from build123d import *

# Parameters (mm, degrees)
EXTRUDE_2_DEPTH = 36


with BuildPart() as part:
    # Эскиз2 → Повернуть1 (revolve)
    with BuildSketch(Plane(origin=(0, 0, 0), x_dir=(1, 0, 0), z_dir=(0, 1, 0))):
        with BuildLine():
            Line((-18, 25), (-18, 0))
            Line((-18, 0), (-20.75, 0))
            Line((-20.75, 0), (-20.75, -2.75))
            Line((-20.75, -2.75), (-18, -2.75))
            Line((-18, -2.75), (-18, -5.5))
            Line((-18, -5.5), (-20.75, -5.5))
            Line((-20.75, -5.5), (-20.75, -8.25))
            Line((-20.75, -8.25), (-18.916666667, -8.25))
            Line((-18.916666667, -8.25), (-18.916666667, -11))
            Line((-18.916666667, -11), (-22, -11))
            ThreePointArc((-22, -11), (-25.889087297, -9.389087297), (-27.5, -5.5))
            Line((-27.5, -5.5), (-27.5, 0))
            Line((-27.5, 0), (-30.395, 2.895))
            Line((-30.395, 2.895), (-30.395, 22.105))
            Line((-30.395, 22.105), (-27.5, 25))
            Line((-27.5, 25), (-18, 25))
        make_face()
    revolve(axis=Axis((0, 0, 84.230364838), (0, 0, -1)))


with BuildPart() as body_2:
    # Эскиз3 → Бобышка-Вытянуть2 (new body)
    with BuildSketch(Plane(origin=(0, 0, -25), x_dir=(-1, 0, 0), z_dir=(0, 0, -1))):
        Polygon((0, -31.754264805), (27.5, -15.877132403), (27.5, 15.877132403), (0, 31.754264805), (-27.5, 15.877132403), (-27.5, -15.877132403), align=None)
    extrude(amount=-EXTRUDE_2_DEPTH)


with BuildPart() as part_1:
    add(part.part)

    # Combine 1: intersect body 2
    add(body_2.part, mode=Mode.INTERSECT)


solid = part_1.part
Source: CAD feature listing. Evaluate the final solid. Frame: model axes, mm. A direction names the side the tool comes from. Give positions to 0.01 mm unless a question says otherwise; leave off trailing zeros. Write each loop counter-clockwise with the first axis right and the second up, starting at its lowest first coordinate (ties: lowest second). Pieces come first, ordered by that corner, then holes. Notation, with made-up numbers: M -21,22.5 L 30,22.5 A22 cw 30,37.5 Z; hole C 71,77 d8. An arc over 180 degrees is marked long. Return JSON: item names as keys, results as strings. Group by question number.
1) Ray query, L1, parallel to Z at x = -18, y = 4.5; L2, parallel to X at y = 1, z = -13.5; L3, parallel to Y at x = -6.5, z = -4. Return the intervals inside material, ascending.
2) Set-up query: faces 1 (the face through (-0.2, 28.3, -0.8)), 2 (the face through (-19.8, 6.2, 1.4)). Return all of +Z, -Z, +X, -X, +Y, -Y with unobstructed straight access to the full face (end or side cutting, diameter ignored); none if empty.
3) Draft query along Y for faces 3 (the face through (24.39, 14.321, -24.216)), 4 (the face through (-24.39, -14.321, -24.216)), 5 (the face through (2.343, 17.847, 4.144)), 6 (the face through (2.343, 17.847, -12.325)). Return one class per face: released by +Y, released by -Y, zero draft, split by the parting line, or undercut.
4) Cut plane C-C, the plane z = -1.5. Output: boundary loops of the cut face in (x, y), then the cut area to 3 significant figures.
5) Cut plane B-B, the plane z = -16.5. Output: boundary loops of the cut face in (x, y) (3 decimals), then the cut area to 3 significant figures.
6) First-contact query: pin 1 Ø1 at (x, z) = (1, 6) entering from -Y; pin 2 Ø5 at (x, z) = (-13.5, -18.5) entering from +Y; pin 3 Ø5 at (x, z) = (-13, -11) entering from -Y. Flat tips, straight axial feed; report the tip coordinate or a pass-through.
Data:
{
 "1": {"L1": "z = -25 to 0, 2.75 to 5.5", "L2": "x = -27.5 to -17.97, 17.97 to 27.5", "L3": "y = -28 to -16.79, 16.79 to 28"},
 "2": {"face 1": "+Z, +Y", "face 2": "none"},
 "3": {"face 3": "released by +Y", "face 4": "released by -Y", "face 5": "undercut", "face 6": "undercut"},
 "4": {"outline": "M -27.5,-9.21 A29 ccw -21.72,-19.21 L -5.78,-28.42 A29 ccw 5.78,-28.42 L 21.72,-19.21 A29 ccw 27.5,-9.21 L 27.5,9.21 A29 ccw 21.72,19.21 L 5.78,28.42 A29 ccw -5.78,28.42 L -21.72,19.21 A29 ccw -27.5,9.21 Z; hole C 0,0 d36", "area": "1,510 mm²"},
 "5": {"outline": "M -27.5,-12.946 A30.395 ccw -24.962,-17.343 L -2.538,-30.289 A30.395 ccw 2.538,-30.289 L 24.962,-17.343 A30.395 ccw 27.5,-12.946 L 27.5,12.946 A30.395 ccw 24.962,17.343 L 2.538,30.289 A30.395 ccw -2.538,30.289 L -24.962,17.343 A30.395 ccw -27.5,12.946 Z; hole C 0,0 d36", "area": "1,580 mm²"},
 "6": {"pin 1": "stops at y = -27.49", "pin 2": "stops at y = 25.4", "pin 3": "stops at y = -25.69"}
}
